```python
from build123d import *

# Parameters (mm, degrees)
F1_DEPTH = 76.2
F3_D     = 12.7
F5_D     = 12.7


with BuildPart() as f1:
    # F0 (on Front) → F1 (new body)
    with BuildSketch(Plane.XZ):
        Polygon((0, 50.8), (0, 0), (127, 0), (127, 25.4), (76.2, 25.4), (76.2, 50.8), align=None)
    extrude(amount=F1_DEPTH)

    # F3 (through all)
    with Locations(Plane.YZ.offset(76.2)):
        with Locations((-38.78307, 37.189245)):
            Hole(F3_D / 2)

    # F5 (through all)
    with Locations(Plane.XY.offset(50.8)):
        with Locations((37.188999, -36.756281)):
            Hole(F5_D / 2)


solid = f1.part
```
Input: part model. Units: mm. Frame: model coordinates. A direction names the side the tool comes from. Give positions to 0.01 mm unless a question says otherwise; leave off trailing zeros. Order: outer loops, then holes, each group sorted by start corner. A loop starts at its lowest first (then second) coordinate and runs counter-clockwise, first axis right, second up.
1. Set-up query: faces 1 (the face through (48, -76.2, 20)), 2 (the face through (102, -38, 25.4)). Return all of +Z, -Z, +X, -X, +Y, -Y with unobstructed straight access to the full face (end or side cutting, diameter ignored); none if empty.
Computed:
face 1: +Z, -Z, +X, -X, -Y
face 2: +Z, +X, +Y, -Y
2. Cut plane D-D (x = 96). Return loops of the section in (y, z), and give its area (3 significant figures).
Computed:
outline: (-76.2, 0) - (0, 0) - (0, 25.4) - (-76.2, 25.4) - close
area: 1,940 mm2
3. Line query: probe 1 along Z at (x, y) = (97.5, -4.5); probe 2 along X at (y, z) = (-26.5, 41); probe 3 along Z at (x, y) = (9, -42.5). Output: solid intervals per line, ascending.
Computed:
probe 1: z = 0 to 25.4
probe 2: x = 0 to 76.2
probe 3: z = 0 to 32.04, 42.34 to 50.8
4. Pin query (flat end, axial travel): pin 1 Ø6 at (x, y) = (38, -38.5) entering from +Z; pin 2 Ø20.5 at (y, z) = (-56.5, 41) entering from +X. Return the tip coordinate at first contact, or that it passes through.
Computed:
pin 1: passes through
pin 2: stops at x = 76.2
5. Cut plane C-C (y = -49). Return loops of the section in (x, z).
Computed:
outline: (0, 0) - (127, 0) - (127, 25.4) - (76.2, 25.4) - (76.2, 50.8) - (0, 50.8) - close
6. Draft query along X for faces 3 (the face through (127, -38, 13)), 4 (the face through (38.02, -30.46, 25.04)), 5 (the face through (48, 0, 20)), 6 (the face through (0, -38, 26)). Return one class per face: released by +X, released by -X, zero draft, split by the parting line, or undercut.
Computed:
face 3: released by +X
face 4: undercut
face 5: zero draft
face 6: released by -X
7. Cut plane A-A (z = 32.5). Return loops of the section in (x, y), and give its area (3 significant figures).
Computed:
outline: (0, -76.2) - (76.2, -76.2) - (76.2, -43.06) - (37.91, -43.06) arc R6.35 cw to (36.46, -43.06) - (0, -43.06) - close; (0, -34.5) - (31.25, -34.5) arc R6.35 cw to (43.13, -34.5) - (76.2, -34.5) - (76.2, 0) - (0, 0) - close
area: 5,120 mm2
8. Cut plane B-B (x = 45). Return loops of the section in (y, z), and give its area (3 significant figures).
Computed:
outline: (-76.2, 0) - (0, 0) - (0, 50.8) - (-76.2, 50.8) - close; hole circle Ø12.7 at (-38.78, 37.19)
area: 3,740 mm2
